Autodesk Inventor part; units mm, degrees
ref_plane "YZ Plane" through (0, 0, 0) normal (1, 0, 0) x (0, 1, 0)
ref_plane "XZ Plane" through (0, 0, 0) normal (0, 1, 0) x (-1, 0, 0)
ref_plane "XY Plane" through (0, 0, 0) normal (0, 0, 1) x (1, 0, 0)
sketch "Sketch1" plane through (0, 0, 0) normal (0, 0, 1) x (1, 0, 0)
  line L0 (-50, 45) -> (50, 45)
  line L1 (50, 45) -> (50, -45)
  line L2 (50, -45) -> (-50, -45)
  line L3 (-50, -45) -> (-50, 45)
  line L4 (-50, -45) -> (50, 45) construction
  point P0 (0, 0)
  point P1 (0, 0)
  dimension "d0" = 100
  dimension "d1" = 90
extrude "Extrusion1" add sketch "Sketch1" along normal blind 2
sketch "Sketch2" plane through (0, 0, 2) normal (0, 0, 1) x (1, 0, 0)
  circle A0 centre (39.0346, -33.2431) radius 1.25
  circle A1 centre (5.1346, -33.2431) radius 1.25
  circle A2 centre (5.1346, 11.6569) radius 1.25
  circle A3 centre (39.0346, 11.6569) radius 1.25
  circle A4 centre (-13.3759, -32.147) radius 1.325
  circle A5 centre (-36.4259, -32.147) radius 1.325
  circle A6 centre (-13.3759, 25.903) radius 1.325
  circle A7 centre (-36.4259, 25.903) radius 1.325
  circle A8 centre (39.0346, -33.2431) radius 1
  circle A9 centre (5.1346, -33.2431) radius 1
  circle A10 centre (-13.3759, -32.147) radius 1
  circle A11 centre (-36.4259, -32.147) radius 1
  circle A12 centre (-13.3759, 25.903) radius 1
  circle A13 centre (-36.4259, 25.903) radius 1
  circle A14 centre (5.1346, 11.6569) radius 1
  circle A15 centre (39.0346, 11.6569) radius 1
  point P0 (0, 0)
  dimension "d4" = 2
  dimension "d5" = 2
  dimension "d6" = 2
  dimension "d7" = 2
  dimension "d8" = 2
  dimension "d9" = 2
  dimension "d10" = 2
  dimension "d11" = 2
extrude "Extrusion2" cut sketch "Sketch2" against normal blind 10 contours A8 | A10 | A13 | A14
sketch "Sketch3" plane through (0, 0, 2) normal (0, 0, 1) x (1, 0, 0)
  circle A0 centre (39.0346, 11.6569) radius 1.25
  circle A1 centre (5.1346, -33.2431) radius 1.25
  circle A2 centre (-36.4259, -32.147) radius 1.325
  circle A3 centre (-13.3759, 25.903) radius 1.325
  circle A4 centre (5.1346, -33.2431) radius 1.1
  circle A5 centre (-36.4259, -32.147) radius 1.175
  circle A6 centre (-13.3759, 25.903) radius 1.175
  circle A7 centre (39.0346, 11.6569) radius 1.1
  point P0 (0, 0)
  dimension "d14" = 0.15
  dimension "d15" = 0.15
  dimension "d16" = 0.15
  dimension "d17" = 0.15
extrude "Extrusion3" add sketch "Sketch3" along normal blind 5 contours A4 | A5 | A6 | A7
equation "\"d15\" = d14"
equation "\"d16\" = d14"
equation "\"d17\" = d14"
properties part number "Electrical Box"
Read the model definition and answer for the solid it produces. Units are mm, in the model's axes. A direction names the side the tool comes from. Round coordinates to 2 decimals unless told otherwise and drop trailing zeros. Write each loop counter-clockwise with the first axis right and the second up, starting at its lowest first coordinate (ties: lowest second). Pieces come first, ordered by that corner, then holes. Notation, with made-up numbers: (38.5, 46.5) - (67.5, 46.5) arc R9 cw to (67.5, 53.5) - close; hole circle Ø9 at (15, 29). An arc over 180 degrees is marked (long way). Use a Markdown table: item, result.
(1) The part is cut by section B-B (z = 3.25). Write down the section's boundary in (x, y) (3 decimals).
Reported:
| item | result |
|---|---|
| outline | circle Ø2.35 at (-36.426, -32.147); circle Ø2.35 at (-13.376, 25.903); circle Ø2.2 at (5.135, -33.243); circle Ø2.2 at (39.035, 11.657) |
(2) The part is cut by section A-A (y = 2.5). Write down the section's boundary in (x, z).
Reported:
| item | result |
|---|---|
| outline | (-50, 0) - (50, 0) - (50, 2) - (-50, 2) - close |
(3) Which of the six approach directions +Z, -Z, +X, -X, +Y, -Y give full straight-line access (tool end or side, diameter ignored) to faces 4 (the cylindrical face through (-14.242, 25.109, 4.465)), 5 (the flat face through (-13, 26, 7))?
Reported:
| item | result |
|---|---|
| face 4 | +Z |
| face 5 | +Z, +X, -X, +Y, -Y |
(4) Straight lines are drawn through the part: line 1 along Z through (x, y) = (-23.5, -1.5); line 2 along X through (y, z) = (12, 3). For each, find the intervals that lie inside material, in ascending order. Write a range as [from, to].
Reported:
| item | result |
|---|---|
| line 1 | [0, 2] |
| line 2 | [37.99, 40.08] |
(5) The part is cut by section C-C (x = 13). Write down the section's boundary in (y, z).
Reported:
| item | result |
|---|---|
| outline | (-45, 0) - (45, 0) - (45, 2) - (-45, 2) - close |
(6) Each of these flat-tipped pins is pushed along its axis until it touches: pin 1 Ø2.5 at (x, y) = (-36.43, 25.9) entering from -Z; pin 2 Ø1.6 at (x, y) = (39.03, -33.24) entering from -Z; pin 3 Ø6 at (x, y) = (10, 20) entering from +Z; pin 4 Ø3 at (x, z) = (-14.5, 5) entering from -Y. Where does it stop, or does it pass through?
Reported:
| item | result |
|---|---|
| pin 1 | z = 0 |
| pin 2 | through |
| pin 3 | z = 2 |
| pin 4 | y = 24.73 |
(7) The mould has two halves that part along X. Classify faces 1 (the flat face through (-1, 1, 0)), 2 (the cylindrical face through (5.642, -32.267, 4.465)), 3 (the cylindrical face through (37.936, 11.609, 4.465)): released by +X, released by -X, zero draft, split by the parting line, or undercut.
Reported:
| item | result |
|---|---|
| face 1 | zero draft |
| face 2 | undercut |
| face 3 | split by the parting line |
